Source: CAD feature listing. Evaluate the final solid. Frame: model axes, mm. A direction names the side the tool comes from. Give positions to 0.01 mm unless a question says otherwise; leave off trailing zeros. Loops run counter-clockwise (first coordinate to the right, second up) from the corner with the lowest first, then second, coordinate; pieces in that order, holes last.
```python
from build123d import *

# Parameters (mm, degrees)
SKETCH1_R               = 8.5
BOSS_EXTRUDE1_DEPTH     = 20
BOSS_EXTRUDE2_DEPTH     = 4
CUT_EXTRUDE1_DEPTH      = 44.400071981
CUT_EXTRUDE1_DEPTH_BACK = 44.400071981
SKETCH3_R               = 5.45
FILLET1_R               = 6


with BuildPart() as part:
    # Sketch1 → Boss-Extrude1 (new, symmetric)
    with BuildSketch(Plane(origin=(0, 0, 0), x_dir=(1, 0, 0), z_dir=(0, 1, 0))):
        with Locations(Location((0, 0, 0), (0, 0, 270))):
            Circle(SKETCH1_R)
    extrude(amount=BOSS_EXTRUDE1_DEPTH, both=True)

    # Sketch2 → Boss-Extrude2 (add, symmetric)
    with BuildSketch(Plane(origin=(0, 0, 0), x_dir=(1, 0, 0), z_dir=(0, 1, 0))):
        Polygon((11.056485774, 6.251996134), (0.113855411, 12.701195624), (-10.942630364, 6.44919949), (-11.056485774, -6.251996134), (-0.113855411, -12.701195624), (10.942630364, -6.44919949), align=None)
    extrude(amount=BOSS_EXTRUDE2_DEPTH, both=True)

    # Sketch3 → Cut-Extrude1 (cut, two sides: drawn at the far end of the back side and taken through both)
    with BuildSketch(Plane(origin=(0, 20, 0), x_dir=(1, 0, 0), z_dir=(0, 1, 0)).offset(-CUT_EXTRUDE1_DEPTH_BACK)):
        with Locations(Location((0, 0, 0), (0, 0, 270))):
            Circle(SKETCH3_R)
    extrude(amount=CUT_EXTRUDE1_DEPTH + CUT_EXTRUDE1_DEPTH_BACK, mode=Mode.SUBTRACT)

    # Fillet1
    # the kernel refuses this fillet: 6 mm, written as the material it takes off along each edge
    with BuildSketch(Plane(origin=(0, -20, 0), x_dir=(0, 0, 1), z_dir=(-1, 0, 0))) as fillet1_piece_1:
        with BuildLine():
            CenterArc((11.45, 5.224700948), FILLET1_R, 180, 60.549814279)
            Line((5.45, 5.224700948), (5.33, 5.224700948))
            Line((5.33, 5.224700948), (5.33, 0))
            Line((5.33, 0), (5.45, -0.12))
            ThreePointArc((5.45, -0.12), (6.975, -0.12), (8.441, -0.104494019))
            Line((8.441, -0.104494019), (8.5, 0))
        make_face()
    revolve(axis=Axis((0, -20, 0), (0, 1, 0)), mode=Mode.SUBTRACT)


solid = part.part
```
(1) First-contact query: pin 1 (2 mm diameter, centred on x = -2, y = -5.5, fed in from +Z); pin 2 (1 mm diameter, centred on y = -2.5, z = -1.5, fed in from +X); pin 3 (4 mm diameter, centred on x = -4, y = -4, fed in from +Z). Flat tips, straight axial feed; report the tip coordinate or a pass-through.
A:
pin 1: stops at z = 8.44
pin 2: stops at x = 11.02
pin 3: stops at z = 11.59
(2) Section C-C, the plane z = 10.75. Return the cut outline in (x, y).
A:
outline: (-3.42, -4) - (3.34, -4) - (3.34, 4) - (-3.42, 4) - close
(3) Section A-A, the plane z = 0. Return the cut outline in (x, y), then the cut area to 3 significant figures.
A:
outline: (-11, -4) - (-8.5, -4) - (-8.5, -20) arc R6 ccw to (-5.45, -14.78) - (-5.45, 20) - (-8.5, 20) - (-8.5, 4) - (-11, 4) - close; (5.45, -14.78) arc R6 ccw to (8.5, -20) - (8.5, -4) - (11, -4) - (11, 4) - (8.5, 4) - (8.5, 20) - (5.45, 20) - close
area: 275 mm2
(4) Section B-B, the plane y = -5. Return the cut outline in (x, z).
A:
outline: circle Ø17 at (0, 0); hole circle Ø10.9 at (0, 0)
(5) Reachability of faces 4 (the flat face through (-5.662, 0.056, 9.431)), 5 (the cylindrical face through (8.428, -11.888, -1.107)), 6 (the flat face through (0, 4, -9)) from +Z, -Z, +X, -X, +Y, -Y: full face, straight path, thin tool, end or side. Return the list, or none.
A:
face 4: +Z, -X, +Y, -Y
face 5: -Y
face 6: +Y
(6) Mould query, pull axis X, two halves, no side actions, for faces 1 (the flat face through (0, -4, -9)), 2 (the cylindrical face through (-5.32, 2.37, -1.18)), 3 (the flat face through (5.662, 0.056, -9.431)). Classes: pulls with the +X half, pulls with the -X half, needs draft (parallel to the pull), parting line crosses it, or undercut.
A:
face 1: needs draft
face 2: undercut
face 3: pulls with the +X half
(7) Ray query, line 1 along X through (y, z) = (7, 0); line 2 along X through (y, z) = (-0.5, -1); line 3 along Y through (x, z) = (1.5, 11). Return the intervals inside material, ascending.
A:
line 1: x = -8.5 to -5.45, 5.45 to 8.5
line 2: x = -10.99 to -5.36, 5.36 to 11.01
line 3: y = -4 to 4
